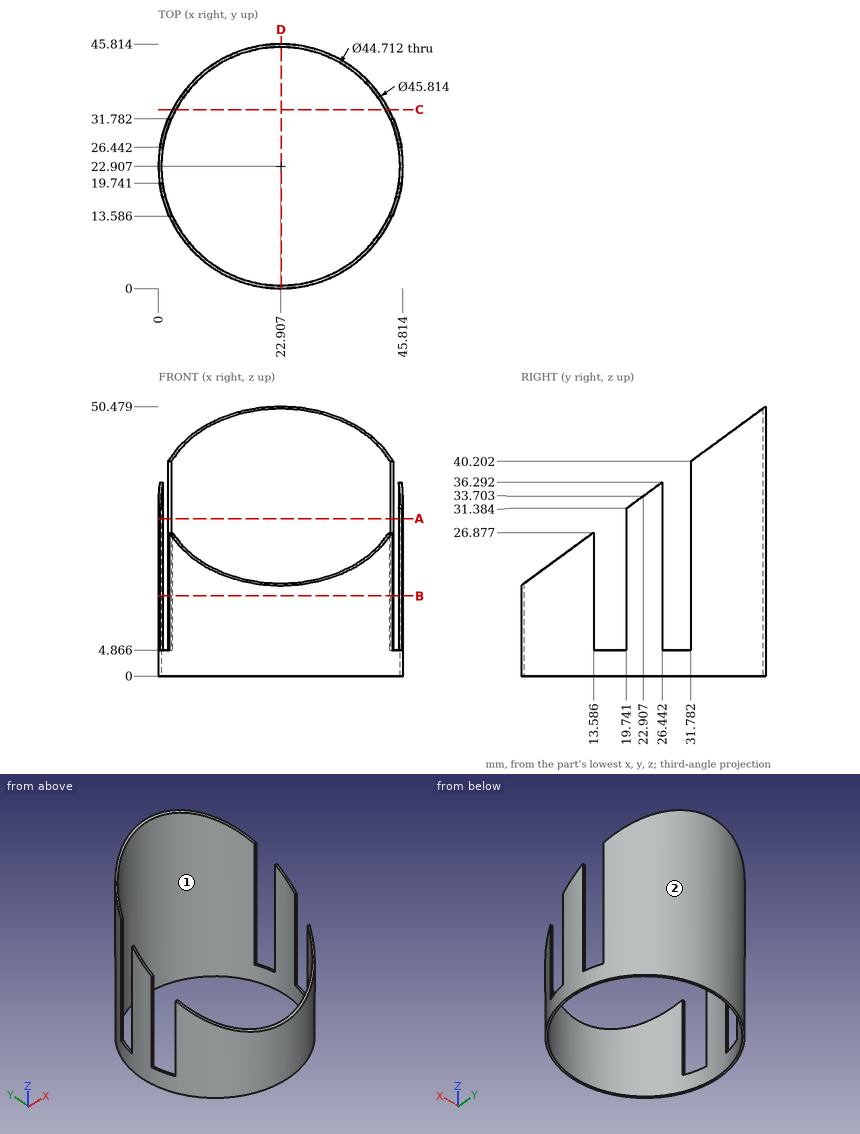
Print and shaded views of the part. All mm, measured from the part's lowest x, y and z. Give positions to 0.01 mm unless a question says otherwise; leave off trailing zeros. Write each loop counter-clockwise with the first axis right and the second up, starting at its lowest first coordinate (ties: lowest second). Pieces come first, ordered by that corner, then holes. Notation, with made-up numbers: (-26, 41.5) - (23, 41.5) arc R3 cw to (23, 46.5) - close; hole circle Ø4 at (81.5, -24). An arc over 180 degrees is marked (long way). Put each result on its own line as item: value.
(1) Pull direction X, two halves, no side cores. Call the marked faces 1 and 2: released by +X, released by -X, zero draft, split by the parting line, or undercut.
Working result:
face 1: undercut
face 2: split by the parting line
(2) Drop flat-ended pins along their axis: pin 1 Ø4 at (x, z) = (31.5, 13) entering from +Y (1 decimal); pin 2 Ø2 at (y, z) = (39.5, 26.5) entering from +X; pin 3 Ø1.9 at (x, y) = (1.5, 18) entering from +Z; pin 4 Ø1.5 at (x, y) = (9.5, 7.5) entering from -Z. Give the stop position or say it passes through.
Working result:
pin 1: y = 44.8
pin 2: x = 39.69
pin 3: z = 4.87
pin 4: through
(3) Saw through at D-D (x = 23). List the corners of the cut face in (y, z) (1 decimal).
Working result:
outline: (0, 0) - (0.6, 0) - (0.6, 17.3) - (0, 16.9) - close; (45.3, 0) - (45.8, 0) - (45.8, 50.5) - (45.3, 50.1) - close
(4) Saw through at B-B (z = 15). List the corners of the cut face in (x, y) (1 decimal).
Working result:
outline: (0.2, 19.7) - (0.8, 19.7) arc R22.4 cw to (0.8, 26.4) - (0.3, 26.4) arc R22.9 ccw to start; (1.8, 31.8) - (2.4, 31.8) arc R22.4 cw to (43.4, 31.8) - (44, 31.8) arc R22.9 ccw to start; (2, 13.6) arc R22.9 ccw to (43.8, 13.6) - (43.2, 13.6) arc R22.4 cw to (2.6, 13.6) - close; (45, 19.7) - (45.6, 19.7) arc R22.9 ccw to (45.5, 26.4) - (45, 26.4) arc R22.4 cw to start
(5) Saw through at C-C (y = 33.5). List the corners of the cut face in (x, z) (1 decimal).
Working result:
outline: (2.6, 0) - (3.2, 0) - (3.2, 41.5) - (2.6, 41.5) - close; (42.6, 0) - (43.2, 0) - (43.2, 41.5) - (42.6, 41.5) - close
(6) Saw through at A-A (z = 29.5). List the corners of the cut face in (x, y) (1 decimal).
Working result:
outline: (0.2, 19.7) - (0.8, 19.7) arc R22.4 cw to (0.8, 26.4) - (0.3, 26.4) arc R22.9 ccw to start; (1.8, 31.8) - (2.4, 31.8) arc R22.4 cw to (43.4, 31.8) - (44, 31.8) arc R22.9 ccw to start; (45, 19.7) - (45.6, 19.7) arc R22.9 ccw to (45.5, 26.4) - (45, 26.4) arc R22.4 cw to start
(7) Wall check: L1, parallel to Y at x = 14, z = 31.5; L2, parallel to X at y = 21, z = 23.5 (1 decimal); L3, parallel to X at y = 38.5, z = 44 (1 decimal). Give the ranges that are in metal, low to high.
Working result:
L1: 43.41 to 44.01
L2: 0.1 to 0.6, 45.2 to 45.7
L3: 6.1 to 6.9, 38.9 to 39.7
